Geometry: final body of the model. Coordinates: model frame, mm. Face numbers are marked on the shaded views. A direction names the side the tool comes from. Round coordinates to 2 decimals unless told otherwise and drop trailing zeros. Loops run counter-clockwise (first coordinate to the right, second up) from the corner with the lowest first, then second, coordinate; pieces in that order, holes last. Notation, with made-up numbers: M 3,-27 L 24,-27 A17 cw 24,-5 Z; hole C 5,-3 d3. An arc over 180 degrees is marked long. Answer as a JSON object with one key per item and string values.
Autodesk Inventor part; units mm, degrees
ref_plane "YZ Plane" through (0, 0, 0) normal (1, 0, 0) x (0, 1, 0)
ref_plane "XZ Plane" through (0, 0, 0) normal (0, 1, 0) x (-1, 0, 0)
ref_plane "XY Plane" through (0, 0, 0) normal (0, 0, 1) x (1, 0, 0)
sketch "Sketch1" plane through (0, 0, 0) normal (0, 1, 0) x (-1, 0, 0)
  line L0 (0, -55.88) -> (-12.7, -55.88)
  line L1 (-12.7, -36.83) -> (0, -36.83)
  line L2 (0, -36.83) -> (0, -55.88)
  line L3 (-12.7, -55.88) -> (-12.7, -36.83)
  dimension "d1" = 19.05
  dimension "d2" = 12.7
extrude "Extrusion1" add sketch "Sketch1" along normal blind 1.5
sketch "Sketch2" plane through (0, 1.5, 0) normal (0, 1, 0) x (1, 0, 0)
  line L0 (12.7, 36.83) -> (12.7, 55.88)
  line L1 (12.7, 0) -> (10.16, 0)
  circle A0 centre (10.16, 39.37) radius 1.092
  circle A1 centre (10.16, 53.34) radius 1.092
  line L2 (10.16, 53.34) -> (10.16, 39.37)
  point P0 (0, 0)
  dimension "d8" = 2.184
  dimension "d10" = 2.184
  dimension "d71" = 13.97
extrude "Extrusion2" cut sketch "Sketch2" against normal blind 1.5
sketch "Sketch5" plane through (0, 0, -36.83) normal (0, 0, 1) x (1, 0, 0)
  line L0 (12.7, 0) -> (0, 0)
  line L1 (6.35, 0) -> (6.35, 1.5)
  line L2 (12.7, 1.5) -> (0, 1.5)
  line L3 (0, 0) -> (0, 1.5)
  line L4 (0, 0.75) -> (12.7, 0.75)
  line L5 (12.7, 0) -> (12.7, 1.5)
  circle A0 centre (6.35, 0.75) radius 5.175
  dimension "d30" = 10.35
extrude "Extrusion5" add sketch "Sketch5" along normal blind 2 contours A0 L0 | L0 L1 L4 A0 | L0 A0 L4 L1 | L4 L1 L2 A0 | L4 A0 L2 L1 | L2 A0
sketch "Sketch6" plane through (6.35, 0.75, -34.83) normal (0, 0, 1) x (1, 0, 0)
  circle A0 centre (0, 0) radius 5.175
  circle A1 centre (0, 0) radius 3.175
  point P0 (-6.35, -0.75)
  dimension "d35" = 6.35
extrude "Extrusion6" add sketch "Sketch6" along normal blind 9
sketch "Sketch7" plane through (12.7, 0, -55.88) normal (0, 0, -1) x (-1, 0, 0)
  line L0 (0, 0) -> (0, 1.5)
  line L1 (0, 0.75) -> (12.7, 0.75)
  line L2 (12.7, 0) -> (12.7, 1.5)
  line L3 (11.4704, 1.5) -> (1.2296, 1.5)
  line L4 (6.35, 1.5) -> (6.35, 0)
  circle A0 centre (6.35, 0.75) radius 5.175
extrude "Extrusion7" add sketch "Sketch7" along normal blind 2
sketch "Sketch8" plane through (6.35, 0.75, -57.88) normal (0, 0, -1) x (-1, 0, 0)
  circle A0 centre (0, 0) radius 5.175
  circle A1 centre (0, 0) radius 3.175
  point P0 (6.35, -0.75)
  dimension "d40" = 6.35
extrude "Extrusion8" add sketch "Sketch8" along normal blind 9
thread "Thread1"
thread "Thread2"
sketch "Sketch9" plane through (0, 0, -36.83) normal (0, 0, -1) x (-1, 0, 0)
  arc A0 (-11.4704, 0) -> (-1.2296, 0) centre (-6.35, 0.75) ccw
  line L0 (0, 0) -> (-1.2296, 0)
  line L1 (-11.4704, 0) -> (-1.2296, 0)
  circle A1 centre (-6.35, 0.75) radius 5.175
extrude "Extrusion9" add sketch "Sketch9" along normal up to next contours L1 A0
sketch "Sketch10" plane through (10.16, 0, -39.37) normal (0, 1, 0) x (1, 0, 0)
  circle A0 centre (0, 0) radius 1.092
  circle A1 centre (0, 13.97) radius 1.092
  circle A2 centre (0, 13.97) radius 1.092
  point P0 (-10.16, -39.37)
  dimension "d60" = 2.184
extrude "Extrusion10" cut sketch "Sketch10" against normal up to next
sketch "Sketch12" plane through (0, 1.5, 0) normal (0, 1, 0) x (1, 0, 0)
  circle A0 centre (10.16, 39.37) radius 1.092
  circle A1 centre (10.16, 39.37) radius 1.092
  circle A2 centre (10.16, 39.37) radius 2.2225
  circle A3 centre (10.16, 53.34) radius 1.092
  circle A4 centre (10.16, 53.34) radius 1.092
  circle A5 centre (10.16, 53.34) radius 2.2225
  point P0 (0, 0)
  dimension "d54" = 4.445
  dimension "d55" = 4.445
extrude "Extrusion11" cut sketch "Sketch12" against normal blind 5.925
sketch "Sketch13" plane through (0, 1.5, 0) normal (0, 1, 0) x (1, 0, 0)
  line L0 (12.7, 36.83) -> (12.7, 55.88)
  line L1 (12.7, 55.88) -> (0, 55.88)
  line L2 (0, 55.88) -> (0, 36.83)
  line L3 (12.7, 36.83) -> (12.7, 55.88)
  circle A0 centre (10.16, 53.34) radius 1.092
  circle A1 centre (10.16, 53.34) radius 1.092
  line L4 (10.16, 53.34) -> (10.16, 39.37)
  circle A2 centre (10.16, 39.37) radius 1.092
  line L5 (0, 36.83) -> (12.7, 36.83)
  point P0 (0, 0)
  point P1 (12.7, 0)
  dimension "d72" = 13.97
  dimension "d73" = 2.184
extrude "Extrusion12" add sketch "Sketch13" along normal blind 10.4775 contours L5 L2 L1 L0 | A2
thread "Thread6"
sketch "Sketch14" plane through (10.16, 1.5, -53.34) normal (0, -1, 0) x (1, 0, 0)
  circle A0 centre (0, 0) radius 1.092
  circle A1 centre (0, 0) radius 2.2225
  circle A2 centre (0, 13.97) radius 2.2225
  circle A3 centre (0, 13.97) radius 2.2225
  circle A4 centre (0, 0) radius 1.092
  circle A5 centre (0, 13.97) radius 1.092
  point P0 (-10.16, 53.34)
extrude "Extrusion13" cut sketch "Sketch14" against normal blind 1
sketch "Sketch15" plane through (10.16, 1.5, -39.37) normal (0, -1, 0) x (1, 0, 0)
  circle A0 centre (0, 0) radius 1.092
  point P0 (-10.16, 39.37)
extrude "Extrusion14" cut sketch "Sketch15" against normal through all
thread "Thread7"
sketch "Sketch16" plane through (0, 11.9775, 0) normal (0, 1, 0) x (1, 0, 0)
  line L0 (11.525, 36.83) -> (1.175, 36.83)
  line L1 (3.175, 34.83) -> (9.525, 34.83)
  line L2 (1.921, 36.83) -> (6.461, 36.83)
  line L3 (6.461, 36.83) -> (6.961, 36.83)
  line L4 (6.961, 36.83) -> (6.961, 39.854)
  line L5 (6.961, 39.854) -> (1.421, 39.854)
  line L6 (1.421, 39.854) -> (1.421, 36.83)
  line L7 (1.421, 36.83) -> (1.921, 36.83)
  point P0 (0, 0)
  point P1 (0, 36.83)
  point P2 (1.2296, 36.83)
  point P3 (11.4704, 36.83)
  dimension "d114" = 0.5
  dimension "d115" = 3.024
  dimension "d116" = 5.54
extrude "Extrusion15" cut sketch "Sketch16" against normal blind 5
sketch "Sketch17" plane through (0, 11.9775, 0) normal (0, 1, 0) x (1, 0, 0)
  line L0 (12.7, 36.83) -> (12.7, 55.88)
  line L1 (12.7, 55.88) -> (0, 55.88)
  line L2 (0, 36.83) -> (12.7, 36.83)
  line L3 (0, 36.83) -> (12.7, 36.83)
  line L4 (12.7, 36.83) -> (12.7, 55.88)
  line L5 (12.7, 55.88) -> (0, 55.88)
  line L6 (0, 55.88) -> (0, 36.83)
  line L7 (11.4704, 41.1651) -> (11.4704, 51.5449)
  line L8 (11.43, 42.545) -> (12.43, 42.545) construction
  line L9 (11.43, 50.165) -> (12.43, 50.165) construction
  line L10 (12.7, 41.545) -> (12.7, 51.165)
  line L11 (12.7, 41.545) -> (12.7, 41.045)
  line L12 (12.7, 41.045) -> (9.93, 41.045)
  line L13 (9.93, 41.045) -> (9.93, 51.665)
  line L14 (9.93, 51.665) -> (12.7, 51.665)
  line L15 (12.7, 51.165) -> (12.7, 51.665)
  point P0 (0, 0)
  dimension "d110" = 2.77
  dimension "d111" = 10.62
  dimension "d112" = 90
extrude "Extrusion16" cut sketch "Sketch17" against normal blind 8 contours L12 L13 L14 L0
properties part number "Line Sensor 6 Bracket"
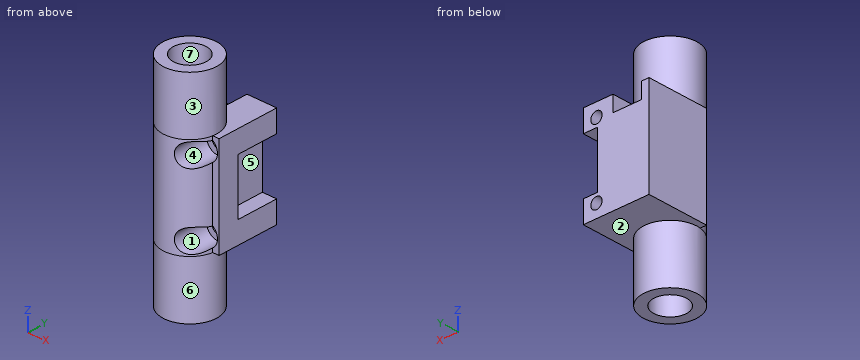
1) Section query D-D (x = 8.5). Return the cut outline in (y, z).
Results:
{"outline": "M -3.96,-66.88 L -1.59,-66.88 L -1.59,-57.88 L 3.09,-57.88 L 3.09,-66.88 L 5.46,-66.88 L 5.46,-55.88 L 11.98,-55.88 L 11.98,-36.83 L 5.46,-36.83 L 5.46,-25.83 L 3.09,-25.83 L 3.09,-34.83 L -1.59,-34.83 L -1.59,-25.83 L -3.96,-25.83 L -3.96,-37.89 L 2.5,-37.89 L 2.5,-40.85 L -3.96,-40.85 L -3.96,-51.86 L 2.5,-51.86 L 2.5,-54.82 L -3.96,-54.82 Z"}
2) Section query C-C (z = -39.37). Return the cut outline in (x, y).
Results:
{"outline": "M 0,0 L 1.23,0 A5.18 ccw 7.94,-4.18 L 7.94,2.5 L 9.07,2.5 L 9.07,11.98 L 6.96,11.98 L 6.96,6.98 L 1.42,6.98 L 1.42,11.98 L 0,11.98 Z; M 11.25,2.5 L 12.38,2.5 L 12.38,0 L 12.7,0 L 12.7,11.98 L 11.25,11.98 Z"}
3) Section query A-A (z = -53.34). Return the cut outline in (x, y).
Results:
{"outline": "M 0,0 L 1.23,0 A5.18 ccw 7.94,-4.18 L 7.94,2.5 L 9.07,2.5 L 9.07,11.98 L 0,11.98 Z; M 11.25,2.5 L 12.38,2.5 L 12.38,0 L 12.7,0 L 12.7,11.98 L 11.25,11.98 Z"}
4) Section query B-B (y = 0.75). Return the cut outline in (x, z) (1 decimal).
Results:
{"outline": "M 0,-55.9 L 1.2,-55.9 L 1.2,-66.9 L 3.2,-66.9 L 3.2,-57.9 L 9.5,-57.9 L 9.5,-66.9 L 11.5,-66.9 L 11.5,-55.9 L 12.7,-55.9 L 12.7,-36.8 L 11.5,-36.8 L 11.5,-25.8 L 9.5,-25.8 L 9.5,-34.8 L 3.2,-34.8 L 3.2,-25.8 L 1.2,-25.8 L 1.2,-36.8 L 0,-36.8 Z; hole C 10.2,-53.3 d4.4; hole C 10.2,-39.4 d4.4"}
5) Reachability of the marked faces 5, 6 and 7 from +Z, -Z, +X, -X, +Y, -Y: full face, straight path, thin tool, end or side. Return the list, or none.
Results:
{"face 5": "+X, +Y", "face 6": "-Z", "face 7": "+Z"}
6) Ray query, line 1 (Z direction, x = 10.16, y = 10.25) (3 decimals); line 2 (Z direction, x = 10.16, y = -1.5); line 3 (Y direction, x = 6.35, z = -63.75) (3 decimals). Return the intervals inside material, ascending.
Results:
{"line 1": "-55.88 to -54.432, -52.248 to -51.665, -41.045 to -40.462, -38.278 to -36.83", "line 2": "-66.88 to -55.56, -51.12 to -41.59, -37.15 to -25.83", "line 3": "-4.425 to -2.425, 3.925 to 5.925"}
7) Pull-direction query (Z, two-part tool) for the marked faces 1, 2, 3 and 4; classes: +Z half, -Z half, draft (parallel to the pull), parting line (faces both ways), or undercut.
Results:
{"face 1": "undercut", "face 2": "-Z half", "face 3": "draft", "face 4": "undercut"}
8) Pin query (flat end, axial travel): P1, Ø6.5, axis at y = 8, z = -44.5, coming from the +X side; P2, Ø1, axis at x = 7, y = 1.5, coming from the +Z side; P3, Ø3.5, axis at x = 10, z = -53, coming from the -Y side. Return the tip coordinate at first contact, or that it passes through.
Results:
{"P1": "x = 9.93", "P2": "z = -34.83", "P3": "y = 2.5"}
